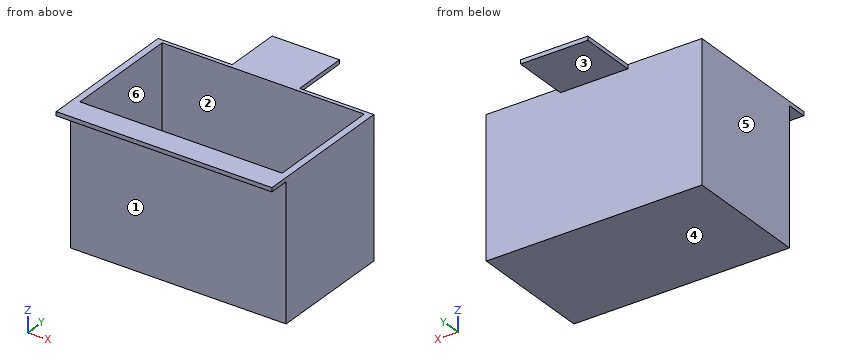
from build123d import *

# Parameters (mm, degrees)
SKETCH_1_W          = 160
SKETCH_1_H          = 150
EXTRUDE_1_DEPTH     = 3
SKETCH_2_W          = 160
SKETCH_2_H          = 92.8
SKETCH_2_W_2        = 150
SKETCH_2_H_2        = 87
EXTRUDE_2_DEPTH     = 100
SKETCH_4_W          = 55
SKETCH_4_H          = 42.2
CUT_EXTRUDE_2_DEPTH = 3
SKETCH_5_W          = 160
SKETCH_5_H          = 15
SKETCH_5_W_2        = 50
SKETCH_5_H_2        = 42.2
EXTRUDE_3_DEPTH     = 3
SKETCH_5_2_W        = 160
SKETCH_5_2_H        = 15
SKETCH_5_2_W_2      = 50
SKETCH_5_2_H_2      = 42.2
CUT_EXTRUDE_3_DEPTH = 149.408220797


with BuildPart() as part:
    # ｽｹｯﾁ1 → ﾎﾞｽ - 押し出し1 (new body)
    with BuildSketch(Plane.XY):
        Rectangle(SKETCH_1_W, SKETCH_1_H)
    extrude(amount=EXTRUDE_1_DEPTH)

    # ｽｹｯﾁ2 → ﾎﾞｽ - 押し出し2 (add)
    with BuildSketch(Plane.XY.offset(3)):
        with Locations((0, -13.6)):
            Rectangle(SKETCH_2_W, SKETCH_2_H)
        with Locations((0, -13.6)):
            Rectangle(SKETCH_2_W_2, SKETCH_2_H_2, mode=Mode.SUBTRACT)
    extrude(amount=EXTRUDE_2_DEPTH)

    # ｽｹｯﾁ4 → ｶｯﾄ - 押し出し2 (cut)
    with BuildSketch(Plane.XY.offset(3)):
        with Locations((-52.5, 53.9)):
            Rectangle(SKETCH_4_W, SKETCH_4_H)
        with Locations((52.5, 53.9)):
            Rectangle(SKETCH_4_W, SKETCH_4_H)
    extrude(amount=-CUT_EXTRUDE_2_DEPTH, mode=Mode.SUBTRACT)

    # ｽｹｯﾁ5 → ﾎﾞｽ - 押し出し3 (add)
    with BuildSketch(Plane(origin=(0, 0, 100), x_dir=(-1, 0, 0), z_dir=(0, 0, -1))):
        with Locations((0, -67.5)):
            Rectangle(SKETCH_5_W, SKETCH_5_H)
        with Locations((0, 53.9)):
            Rectangle(SKETCH_5_W_2, SKETCH_5_H_2)
    extrude(amount=-EXTRUDE_3_DEPTH)

    # ｽｹｯﾁ5<2> → ｶｯﾄ - 押し出し3 (cut, through all)
    with BuildSketch(Plane(origin=(0, 0, 100), x_dir=(-1, 0, 0), z_dir=(0, 0, -1))):
        with Locations((0, -67.5)):
            Rectangle(SKETCH_5_2_W, SKETCH_5_2_H)
        with Locations((0, 53.9)):
            Rectangle(SKETCH_5_2_W_2, SKETCH_5_2_H_2)
    extrude(amount=CUT_EXTRUDE_3_DEPTH, mode=Mode.SUBTRACT)


solid = part.part
Can you work these out from the model? Positions are in its coordinate system, mm. Face numbers are marked on the shaded views. A direction names the side the tool comes from. Coordinates: 2 decimals unless noted, no trailing zeros. Loops run counter-clockwise (first coordinate to the right, second up) from the corner with the lowest first, then second, coordinate; pieces in that order, holes last. Notation, with made-up numbers: M 54,24 L 61,24 A9 ccw 61,35 Z; hole C 31,67.25 d5. An arc over 180 degrees is marked long. Answer as CSV lines item,"result". Start each with the question number.
1. For the marked faces 1, 2 and 3, which set-ups out of +Z, -Z, +X, -X, +Y, -Y let a thin tool reach every point of the face, with its end or its side?
2. Suppose I cut it at D-D, the plane x = -63. List the corners of the cut face in (y, z) for me, plus the area to 3 significant figures.
3. If I drill on probe 1 along Y at (x, z) = (-43.5, 74); probe 2 along X at (y, z) = (28.5, 87); probe 3 along Z at (x, y) = (67, -40.5), over which ranges is the centre line in solid material (lowest first)? Write a range as [from, to].
4. Suppose I cut it at C-C, the plane y = 21. List the corners of the cut face in (x, z) for me.
5. For pin 1 Ø1 at (x, z) = (7, 37.5) entering from +Y; pin 2 Ø12 at (x, y) = (7.5, -44) entering from +Z; pin 3 Ø0.9 at (y, z) = (45, 102) entering from +X, each with a flat end and sliding along its axis, tell me the tip position at first contact or that it passes through.
6. Suppose I cut it at B-B, the plane x = 4. List the corners of the cut face in (y, z) for me, plus the area to 3 significant figures.
7. Suppose I cut it at A-A, the plane z = 19. List the corners of the cut face in (x, y) for me, plus the area to 3 significant figures.
8. Thinking about a two-plate mould opening in X: for the marked faces 4, 5 and 6, which applies, +X half, -X half, draft (parallel to the pull), parting line (faces both ways), or undercut?
Output:
1,face 1,"-Z, +X, -X, -Y"
1,face 2,"+Z"
1,face 3,"-Z, +X, -X, +Y"
2,outline,"M -75,100 L -60,100 L -60,0 L 32.8,0 L 32.8,103 L 29.9,103 L 29.9,3 L -57.1,3 L -57.1,103 L -75,103 Z"
2,area,"903 mm^2"
3,probe 1,"y = [-60, -57.1], [29.9, 32.8]"
3,probe 2,"x = [-80, -75], [75, 80]"
3,probe 3,"z = [0, 3]"
4,outline,"M -80,0 L 80,0 L 80,103 L 75,103 L 75,3 L -75,3 L -75,103 L -80,103 Z"
5,pin 1,"stops at y = 32.8"
5,pin 2,"stops at z = 3"
5,pin 3,"stops at x = 25"
6,outline,"M -75,100 L -60,100 L -60,0 L 32.8,0 L 32.8,100 L 75,100 L 75,103 L 29.9,103 L 29.9,3 L -57.1,3 L -57.1,103 L -75,103 Z"
6,area,"1,030 mm^2"
7,outline,"M -80,-60 L 80,-60 L 80,32.8 L -80,32.8 Z; hole M -75,-57.1 L 75,-57.1 L 75,29.9 L -75,29.9 Z"
7,area,"1,800 mm^2"
8,face 4,"draft"
8,face 5,"-X half"
8,face 6,"undercut"
